from build123d import *

# Parameters (mm, degrees)
F1_DEPTH = 30
F2_R     = 22.490122
F3_DEPTH = 30.001


with BuildPart() as f1:
    # F0 (on Top) → F1 (new body)
    with BuildSketch(Plane.XY):
        with BuildLine():
            ThreePointArc((0, 40), (-28.284271, -28.284271), (40, 0))
            ThreePointArc((40, 0), (28.284271, 28.284271), (0, 40))
        make_face()
    extrude(amount=F1_DEPTH)

    # F2 (on face) → F3 (cut, through all)
    with BuildSketch(Plane.XY.offset(30)):
        Circle(F2_R)
    extrude(amount=-F3_DEPTH, mode=Mode.SUBTRACT)


with BuildPart() as f4_1:
    # F4: copy of F1
    add(f1.part)


solid = f1.part
Verification items for the finished model (mm, model axes). Give positions to 0.01 mm unless a question says otherwise; leave off trailing zeros. Write each loop counter-clockwise with the first axis right and the second up, starting at its lowest first coordinate (ties: lowest second). Pieces come first, ordered by that corner, then holes. Notation, with made-up numbers: M 19,61.5 L 72,61.5 A18 cw 72,88.5 Z; hole C -31.75,67 d11. An arc over 180 degrees is marked long. Put each result on its own line as item: value. Start each with the question number.
1. Section check A-A (y = 15). Record the cut outline in (x, z).
2. Go/stop test with flat-tipped pins: pin 1 Ø8 at (x, z) = (-26, 25) entering from +Y; pin 2 Ø4 at (x, z) = (21, 14.5) entering from +Y; pin 3 Ø1 at (y, z) = (-4, 14.5) entering from +X. Record where each tip stops, or that it passes through.
3. Section check B-B (x = -8). Record the cut outline in (y, z).
4. Scan lines: line 1 along X through (y, z) = (0.5, 28); line 2 along Y through (x, z) = (0, 20.5); line 3 along X through (y, z) = (4, 10). Record each from-to range of solid material in increasing order. Write a range as [from, to].
5. Section check C-C (z = 6.25). Record the cut outline in (x, y).
6. Section check D-D (x = -29). Record the cut outline in (y, z), and give its area (3 significant figures).
7. Draft check along X on faces 1 (the face through (21.45, 6.76, 15.21)), 2 (the face through (17, -17, 0)). Enter one of: +X half, -X half, draft (parallel to the pull), parting line (faces both ways), or undercut.
Answer list:
1. outline: M -37.08,0 L -16.76,0 L -16.76,30 L -37.08,30 Z; M 16.76,0 L 37.08,0 L 37.08,30 L 16.76,30 Z
2. pin 1: y = 33.41
2. pin 2: y = 35.2
2. pin 3: x = 39.85
3. outline: M -39.19,0 L -21.02,0 L -21.02,30 L -39.19,30 Z; M 21.02,0 L 39.19,0 L 39.19,30 L 21.02,30 Z
4. line 1: [-40, -22.48], [22.48, 40]
4. line 2: [-40, -22.49], [22.49, 40]
4. line 3: [-39.8, -22.13], [22.13, 39.8]
5. outline: C 0,0 d80; hole C 0,0 d44.98
6. outline: M -27.55,0 L 27.55,0 L 27.55,30 L -27.55,30 Z
6. area: 1,650 mm2
7. face 1: undercut
7. face 2: draft
